from build123d import *

# Parameters (mm, degrees)
F1_DEPTH = 63.5
F0_W     = 25.4
F0_H     = 19.05
F2_DEPTH = 25.4
F3_DEPTH = 7.9375
F5_R     = 5.08


with BuildPart() as f1:
    # F0 (on Front) → F1 (new body, symmetric)
    with BuildSketch(Plane.XZ):
        Polygon((22.225, 9.525), (-41.275, 9.525), (-41.275, -9.525), (41.275, -9.525), (41.275, 9.525), align=None)
    extrude(amount=F1_DEPTH, both=True)

    # F0 (on Front) → F2 (join, symmetric)
    with BuildSketch(Plane.XZ):
        with Locations((73.025, 52.4002)):
            Rectangle(F0_W, F0_H)
        with BuildLine():
            Line((22.225, 30.1469992557), (22.225, 9.525))
            Line((22.225, 9.525), (41.275, 9.525))
            Line((41.275, 9.525), (41.275, 29.1625964248))
            ThreePointArc((41.275, 29.1625964248), (46.4882785135, 38.9596049457), (56.8722933531, 42.8752))
            Line((56.8722933531, 42.8752), (60.325, 42.8752))
            Line((60.325, 42.8752), (60.325, 61.9252))
            Line((60.325, 61.9252), (56.8722933531, 61.9252))
            ThreePointArc((56.8722933531, 61.9252), (33.3654380804, 52.7775587752), (22.225, 30.1469992557))
        make_face()
    extrude(amount=F2_DEPTH, both=True)

    # F0 (on Front) → F3 (join, symmetric)
    with BuildSketch(Plane.XZ):
        with BuildLine():
            add(Edge.make_bspline(
                [(-41.275, 9.525), (-41.275, 37.3456478119), (0, 61.9252), (56.8722933531, 61.9252)],
                knots=[0, 0, 0, 0, 111.2594811806, 111.2594811806, 111.2594811806, 111.2594811806], degree=3))
            Line((-41.275, 9.525), (22.225, 9.525))
            Line((22.225, 9.525), (22.225, 30.1469992557))
            ThreePointArc((22.225, 30.1469992557), (33.3654380804, 52.7775587752), (56.8722933531, 61.9252))
        make_face()
    extrude(amount=F3_DEPTH, both=True)

    # F0 (on Front) → F4 (revolve)
    with BuildSketch(Plane.XZ):
        Polygon((85.725, 66.675), (85.725, 61.9252), (85.725, 42.8752), (85.725, 38.1), (111.125, 38.1), (111.125, 66.675), align=None)
    revolve(axis=Axis((85.725, 0, 52.3875), (0, 0, 1)))

    # F5
    f5_edges = [f1.edges().sort_by_distance(p)[0] for p in [
        (-41.275, -63.5, 0),
        (41.275, -63.5, 0),
        (41.275, 63.5, 0),
        (-41.275, 63.5, 0),
    ]]
    fillet(f5_edges, radius=F5_R)


solid = f1.part
Geometry: final body of the model. Coordinates: model frame, mm. A direction names the side the tool comes from. Give positions to 0.01 mm unless a question says otherwise; leave off trailing zeros. Write each loop counter-clockwise with the first axis right and the second up, starting at its lowest first coordinate (ties: lowest second). Pieces come first, ordered by that corner, then holes. Notation, with made-up numbers: (-11, 18) -> (2, 18) arc R28 ccw to (2, 55) -> close; hole circle Ø8 at (-14, 71.25). An arc over 180 degrees is marked (long way). Answer as a JSON object with one key per item and string values.
1. Access query for faces 4 (the cylindrical face through (33.63, -16.79, 53.02)), 5 (the flat face through (59, 0, 42.875)), 6 (the flat face through (46, -25.4, 42)). Directions: +Z, -Z, +X, -X, +Y, -Y. A direction counts if a zero-diameter tool reaches every point of the face in a straight line with its end or side. Return the directions, or none.
Ans:
{"face 4": "+Z, -X, -Y", "face 5": "-Z", "face 6": "+Z, +X, -X, -Y"}
2. Cut plane B-B on x = 78. Output: boundary loops of the cut face in (y, z) (3 decimals).
Ans:
{"outline": "(-25.4, 42.875) -> (-24.197, 42.875) -> (-24.197, 38.1) -> (24.197, 38.1) -> (24.197, 42.875) -> (25.4, 42.875) -> (25.4, 61.925) -> (24.197, 61.925) -> (24.197, 66.675) -> (-24.197, 66.675) -> (-24.197, 61.925) -> (-25.4, 61.925) -> close"}
3. Ray query, probe 1 along Z at (x, y) = (-16, -16.5) (3 decimals); probe 2 along Y at (x, z) = (36, 33); probe 3 along Z at (x, y) = (81.5, 11.5) (3 decimals). Return the intervals inside material, ascending. Write a range as from..to.
Ans:
{"probe 1": "z = -9.525..9.525", "probe 2": "y = -25.4..25.4", "probe 3": "z = 38.1..66.675"}
4. Mould query, pull axis X, two halves, no side actions, for faces 1 (the cylindrical face through (33.63, 16.55, 53.02)), 2 (the flat face through (1, -36, 9.525)), 3 (the cylindrical face through (46.37, -0.356, 38.854)). Classes: pulls with the +X half, pulls with the -X half, needs draft (parallel to the pull), parting line crosses it, or undercut.
Ans:
{"face 1": "pulls with the -X half", "face 2": "needs draft", "face 3": "undercut"}
5. Cut plane A-A on z = 2. Output: boundary loops of the cut face in (x, y) (3 decimals).
Ans:
{"outline": "(-41.275, -58.42) arc R5.08 ccw to (-36.195, -63.5) -> (36.195, -63.5) arc R5.08 ccw to (41.275, -58.42) -> (41.275, 58.42) arc R5.08 ccw to (36.195, 63.5) -> (-36.195, 63.5) arc R5.08 ccw to (-41.275, 58.42) -> close"}
6. Contact query for flat-ended pins moving along their axis: pin 1 (5 mm diameter, centred on y = 14.5, z = 38.5, fed in from +X); pin 2 (16.5 mm diameter, centred on x = -5, y = 42, fed in from +Z) (3 decimals); pin 3 (11.5 mm diameter, centred on y = -14.5, z = 1.5, fed in from +X) (3 decimals). Output: stop coordinate, or through.
Ans:
{"pin 1": "stops at x = 108.11", "pin 2": "stops at z = 9.525", "pin 3": "stops at x = 41.275"}
7. Cut plane D-D on y = 20. Output: boundary loops of the cut face in (x, z) (3 decimals).
Ans:
{"outline": "(-41.275, -9.525) -> (41.275, -9.525) -> (41.275, 29.163) arc R15.727 cw to (56.872, 42.875) -> (70.067, 42.875) -> (70.067, 38.1) -> (101.383, 38.1) -> (101.383, 66.675) -> (70.067, 66.675) -> (70.067, 61.925) -> (56.872, 61.925) arc R34.777 ccw to (22.225, 30.147) -> (22.225, 9.525) -> (-41.275, 9.525) -> close"}
8. Cut plane C-C on y = -13. Output: boundary loops of the cut face in (x, z) (3 decimals).
Ans:
{"outline": "(-41.275, -9.525) -> (41.275, -9.525) -> (41.275, 29.163) arc R15.727 cw to (56.872, 42.875) -> (63.904, 42.875) -> (63.904, 38.1) -> (107.546, 38.1) -> (107.546, 66.675) -> (63.904, 66.675) -> (63.904, 61.925) -> (56.872, 61.925) arc R34.777 ccw to (22.225, 30.147) -> (22.225, 9.525) -> (-41.275, 9.525) -> close"}
